from build123d import *

# Parameters (mm, degrees)
BOSS_EXTRUDE1_DEPTH = 7.95
SKETCH2_R           = 2.4
BOSS_EXTRUDE2_DEPTH = 1.8
LPATTERN1_COUNT     = 2
LPATTERN1_PITCH     = 8
SHELL1_T            = -0.5
SKETCH3_R           = 3
SKETCH3_R_2         = 2.4
BOSS_EXTRUDE3_DEPTH = 9.1
SKETCH4_W           = 10.998295323
SKETCH4_H           = 15.9
CUT_EXTRUDE1_DEPTH  = 15.757300106


with BuildPart() as part:
    # Sketch1 → Boss-Extrude1 (new, symmetric)
    with BuildSketch(Plane.XY):
        Polygon((0, 0), (-15.9, 0), (-15.9, 2), (-7.95, 9.6), (0, 9.6), align=None)
    extrude(amount=BOSS_EXTRUDE1_DEPTH, both=True)

    # Sketch2 → Boss-Extrude2 (add)
    with BuildSketch(Plane(origin=(0, 9.6, 0), x_dir=(1, 0, 0), z_dir=(0, 1, 0))):
        with Locations(Location((-4.05, -4.05, 0), (0, 0, 270))):
            Circle(SKETCH2_R)
    boss_extrude2 = extrude(amount=BOSS_EXTRUDE2_DEPTH)

    # LPattern1: Boss-Extrude2 ×2
    with Locations(*[(0, 0, -i * LPATTERN1_PITCH) for i in range(1, LPATTERN1_COUNT)]):
        add(boss_extrude2)

    # Shell1
    shell1_openings = [part.faces().sort_by_distance(p)[0] for p in [
        (-7.95, 0, 0),
    ]]
    offset(amount=SHELL1_T, openings=shell1_openings, kind=Kind.INTERSECTION)

    # Sketch3 → Boss-Extrude3 (add)
    with BuildSketch(Plane.XZ.offset(-9.1)):
        with Locations(Location((-8.05, 0.05, 0), (0, 0, 84.250353958))):
            Circle(SKETCH3_R)
        with Locations(Location((-8.05, 0.05, 0), (0, 0, 82.806112334))):
            Circle(SKETCH3_R_2, mode=Mode.SUBTRACT)
    extrude(amount=BOSS_EXTRUDE3_DEPTH)

    # Sketch4 → Cut-Extrude1 (cut, through all)
    with BuildSketch(Plane(origin=(-8.591290689, 8.986942234, 0), x_dir=(0.7228392916279055, 0.6910161781600108, 0), z_dir=(-0.6910161781600108, 0.7228392916279055, 0))):
        with Locations((-4.611964719, 0)):
            Rectangle(SKETCH4_W, SKETCH4_H)
    extrude(amount=CUT_EXTRUDE1_DEPTH, mode=Mode.SUBTRACT)


solid = part.part
Check sheet for the modelled part. Datum: model origin and axes. Units: mm. A direction names the side the tool comes from. Give positions to 0.01 mm unless a question says otherwise; leave off trailing zeros. Loops run counter-clockwise (first coordinate to the right, second up) from the corner with the lowest first, then second, coordinate; pieces in that order, holes last. Notation, with made-up numbers: M 51.5,75 L 90.5,75 A10 ccw 90.5,88 Z; hole C 52,-22.5 d8. An arc over 180 degrees is marked long. Answer as a JSON object with one key per item and string values. Group by question number.
Q1. Access from +Z, -Z, +X, -X, +Y, -Y to the whole of each face (thin tool, end or side, straight path). Record for faces 1 (the cylindrical face through (-5.8, 4.61, 0.88)), 2 (the flat face through (-4, 11.4, 4)).
Q2. Cross-section at D-D on y = 3. Record the cut outline in (x, z), then the cut area to 3 significant figures.
Q3. Material ranges on line 1 along Z through (x, y) = (-8.05, 5.25); line 2 along X through (y, z) = (9.9, -3.95); line 3 along Z through (x, y) = (-5, 8.75), recorded low to high. Write a range as [from, to].
Q4. Cross-section at C-C on z = -3.95. Record the cut outline in (x, y).
Q5. Go/stop test with flat-tipped pins: P1, Ø2, axis at x = -12.5, z = 4, coming from the +Y side; P2, Ø6, axis at x = -4.5, y = 10, coming from the +Z side; P3, Ø2.5, axis at x = -4.05, z = 4.05, coming from the -Y side; P4, Ø3.5, axis at x = -3.5, z = -1.5, coming from the -Y side. Record where each tip stops, or that it passes through.
Q6. Cross-section at B-B on x = -4.05. Record the cut outline in (y, z), then the cut area to 4 significant figures.
Q7. Release check for a two-part mould opening along X. For faces 3 (the flat face through (-4, 9.6, 0)), 4 (the cylindrical face through (-6.18, 10.49, 5.16)), 5 (the flat face through (-8.819, 8.078, 0.084)) record: released by +X, released by -X, zero draft, split by the parting line, or undercut.
Q8. Cross-section at A-A on y = 1. Record the cut outline in (x, z).
Evaluation:
{
 "1": {"face 1": "-Y", "face 2": "+Z, -Z, +X, -X, +Y"},
 "2": {"outline": "M -14.85,-7.95 L 0,-7.95 L 0,7.95 L -14.85,7.95 Z; C -8.05,0.05 d6; hole M -14.13,-7.45 L -0.5,-7.45 L -0.5,7.45 L -14.13,7.45 Z; hole C -8.05,0.05 d4.8", "area": "43.3 mm2"},
 "3": {"line 1": "z = [-7.95, -7.45], [-2.95, -2.35], [2.45, 3.05], [7.45, 7.95]", "line 2": "x = [-6.45, -5.95], [-2.15, -1.65]", "line 3": "z = [-7.95, -7.45], [7.45, 7.95]"},
 "4": {"outline": "M -15.9,0 L -15.4,0 L -15.4,1.79 L -7.75,9.1 L -5.95,9.1 L -5.95,10.9 L -2.15,10.9 L -2.15,9.1 L -0.5,9.1 L -0.5,0 L 0,0 L 0,9.6 L -1.65,9.6 L -1.65,11.4 L -6.45,11.4 L -6.45,9.6 L -7.95,9.6 L -15.9,2 Z"},
 "5": {"P1": "stops at y = 6.21", "P2": "stops at z = 7.95", "P3": "stops at y = 10.9", "P4": "stops at y = 9.1"},
 "6": {"outline": "M 0,-7.95 L 9.6,-7.95 L 9.6,-6.35 L 11.4,-6.35 L 11.4,-1.55 L 9.6,-1.55 L 9.6,1.65 L 11.4,1.65 L 11.4,6.45 L 9.6,6.45 L 9.6,7.95 L 0,7.95 L 0,7.45 L 9.1,7.45 L 9.1,5.95 L 10.9,5.95 L 10.9,2.15 L 9.1,2.15 L 9.1,-2.05 L 10.9,-2.05 L 10.9,-5.85 L 9.1,-5.85 L 9.1,-7.45 L 0,-7.45 Z", "area": "20.65 mm2"},
 "7": {"face 3": "zero draft", "face 4": "split by the parting line", "face 5": "undercut"},
 "8": {"outline": "M -15.9,-7.95 L 0,-7.95 L 0,7.95 L -15.9,7.95 Z; C -8.05,0.05 d6; hole M -15.4,-7.45 L -0.5,-7.45 L -0.5,7.45 L -15.4,7.45 Z; hole C -8.05,0.05 d4.8"}
}
